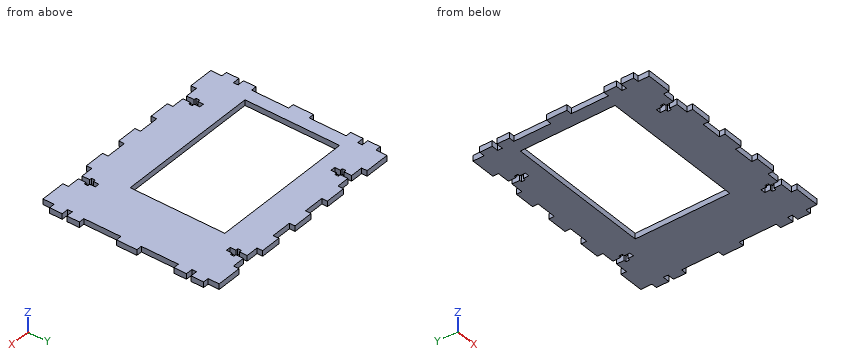
```python
from build123d import *

# Parameters (mm, degrees)
SKETCH004_W                   = 120
SKETCH004_H                   = 95
PAD001_DEPTH                  = 3
SKETCH005_W                   = 3
SKETCH005_H                   = 6
SKETCH005_H_2                 = 20
SKETCH005_W_2                 = 16
SKETCH005_H_3                 = 3
SKETCH005_W_3                 = 11
POCKET003_DEPTH               = 309.164355
SKETCH005_MIRRORED006_2_W     = 3
SKETCH005_MIRRORED006_2_H     = 6
SKETCH005_MIRRORED006_2_H_2   = 20
SKETCH005_MIRRORED006_2_W_2   = 16
SKETCH005_MIRRORED006_2_H_3   = 3
SKETCH005_MIRRORED006_2_W_3   = 11
POCKET003_MIRRORED006_2_DEPTH = 309.164355
SKETCH006_W                   = 3.7
SKETCH006_H                   = 2.5
POCKET004_DEPTH               = 309.164355
SKETCH006_MIRRORED008_2_W     = 3.7
SKETCH006_MIRRORED008_2_H     = 2.5
POCKET004_MIRRORED008_2_DEPTH = 309.164355
SKETCH007_W                   = 78
SKETCH007_H                   = 51
POCKET005_DEPTH               = 3.001


with BuildPart() as part:
    # Sketch004 → Pad001 (new body)
    with BuildSketch(Plane.XY):
        Rectangle(SKETCH004_W, SKETCH004_H)
    extrude(amount=PAD001_DEPTH)

    # Sketch005 → Pocket003 (cut, through all)
    with BuildSketch(Plane.XY):
        with Locations((-58.5, 44.5)):
            Rectangle(SKETCH005_W, SKETCH005_H)
        with Locations((-58.5, 15.5)):
            Rectangle(SKETCH005_W, SKETCH005_H_2)
        with Locations((-35.5, 46)):
            Rectangle(SKETCH005_W_2, SKETCH005_H_3)
        with Locations((-11, 46)):
            Rectangle(SKETCH005_W_3, SKETCH005_H_3)
    pocket003 = extrude(amount=POCKET003_DEPTH, mode=Mode.SUBTRACT)

    # Sketch005 Mirrored006 2 → Pocket003 Mirrored006 2 (cut, through all)
    with BuildSketch(Plane(origin=(0, 0, 0), x_dir=(-1, 0, 0), z_dir=(0, 0, -1))):
        with Locations((-58.5, 44.5)):
            Rectangle(SKETCH005_MIRRORED006_2_W, SKETCH005_MIRRORED006_2_H)
        with Locations((-58.5, 15.5)):
            Rectangle(SKETCH005_MIRRORED006_2_W, SKETCH005_MIRRORED006_2_H_2)
        with Locations((-35.5, 46)):
            Rectangle(SKETCH005_MIRRORED006_2_W_2, SKETCH005_MIRRORED006_2_H_3)
        with Locations((-11, 46)):
            Rectangle(SKETCH005_MIRRORED006_2_W_3, SKETCH005_MIRRORED006_2_H_3)
    pocket003_mirrored006_2 = extrude(amount=-POCKET003_MIRRORED006_2_DEPTH, mode=Mode.SUBTRACT)

    # Mirrored007: Pocket003, Pocket003 Mirrored006 2 across Sketch005 H_Axis
    add(pocket003.mirror(Plane.ZX), mode=Mode.SUBTRACT)
    add(pocket003_mirrored006_2.mirror(Plane.ZX), mode=Mode.SUBTRACT)

    # Sketch006 → Pocket004 (cut, through all)
    with BuildSketch(Plane.XY):
        with Locations((-58.15, 33.5)):
            Rectangle(SKETCH006_W, SKETCH006_H)
        Polygon((-36.75, 47.5), (-34.25, 47.5), (-34.25, 40.4), (-33, 40.4), (-33, 38.4), (-34.25, 38.4), (-34.25, 35.4), (-36.75, 35.4), (-36.75, 38.4), (-38, 38.4), (-38, 40.4), (-36.75, 40.4), align=None)
    pocket004 = extrude(amount=POCKET004_DEPTH, mode=Mode.SUBTRACT)

    # Sketch006 Mirrored008 2 → Pocket004 Mirrored008 2 (cut, through all)
    with BuildSketch(Plane(origin=(0, 0, 0), x_dir=(-1, 0, 0), z_dir=(0, 0, -1))):
        with Locations((-58.15, 33.5)):
            Rectangle(SKETCH006_MIRRORED008_2_W, SKETCH006_MIRRORED008_2_H)
        Polygon((-36.75, 47.5), (-34.25, 47.5), (-34.25, 40.4), (-33, 40.4), (-33, 38.4), (-34.25, 38.4), (-34.25, 35.4), (-36.75, 35.4), (-36.75, 38.4), (-38, 38.4), (-38, 40.4), (-36.75, 40.4), align=None)
    pocket004_mirrored008_2 = extrude(amount=-POCKET004_MIRRORED008_2_DEPTH, mode=Mode.SUBTRACT)

    # Mirrored009: Pocket004, Pocket004 Mirrored008 2 across Sketch006 H_Axis
    add(pocket004.mirror(Plane.ZX), mode=Mode.SUBTRACT)
    add(pocket004_mirrored008_2.mirror(Plane.ZX), mode=Mode.SUBTRACT)

    # Sketch007 → Pocket005 (cut, through all)
    with BuildSketch(Plane.XY):
        with Locations((-11, 2)):
            Rectangle(SKETCH007_W, SKETCH007_H)
    extrude(amount=POCKET005_DEPTH, mode=Mode.SUBTRACT)


with BuildPart() as part_1:
    # Body001 placement: moved
    add(part.part.moved(Location((0, 0, 38))))


solid = part_1.part
```
Geometry check sheet. Reference: the model listing, model coordinates, mm. Coordinates: 2 decimals unless noted, no trailing zeros. Order: outer loops, then holes, each group sorted by start corner. A loop starts at its lowest first (then second) coordinate and runs counter-clockwise, first axis right, second up. Notation, with made-up numbers: M 65.5,-15.5 L 90.5,-15.5 A35 cw 90.5,22.5 Z; hole C 47,-21 d1. An arc over 180 degrees is marked long. One line per question, with ' | ' between items. Start each with the question number.
Item 1: Cross-section at A-A on x = 2.5. Enter the section's corners in (y, z), then the cut area to 3 significant figures.
Item 2: Material ranges on L1, parallel to X at y = 40, z = 39.95; L2, parallel to Y at x = -28, z = 38.3; L3, parallel to Y at x = -49, z = 38.2, recorded low to high. Write a range as [from, to].
Item 3: Gauge pin test, flat ends, axial feed: pin 1 (1.5 mm diameter, centred on y = -44.5, z = 39, fed in from -X); pin 2 (0.8 mm diameter, centred on y = -34, z = 40, fed in from -X); pin 3 (0.9 mm diameter, centred on x = 58.5, z = 39, fed in from -Y). Record the tip position at first contact, or that the pin passes through.
Item 4: Cross-section at B-B on y = 24. Enter the section's corners in (x, z), then the cut area to 3 significant figures.
Findings:
1) outline: M -47.5,38 L -23.5,38 L -23.5,41 L -47.5,41 Z; M 27.5,38 L 47.5,38 L 47.5,41 L 27.5,41 Z | area: 132 mm²
2) L1: x = [-60, -38], [-33, 33], [38, 60] | L2: y = [-44.5, -23.5], [27.5, 44.5] | L3: y = [-47.5, -23.5], [27.5, 47.5]
3) pin 1: stops at x = -57 | pin 2: stops at x = -56.3 | pin 3: stops at y = -41.5
4) outline: M -57,38 L -50,38 L -50,41 L -57,41 Z; M 28,38 L 57,38 L 57,41 L 28,41 Z | area: 108 mm²
